Can you work these out from the model? Positions are in its coordinate system, mm. Give positions to 0.01 mm unless a question says otherwise; leave off trailing zeros. Loops run counter-clockwise (first coordinate to the right, second up) from the corner with the lowest first, then second, coordinate; pieces in that order, holes last. Notation, with made-up numbers: M 65.25,79 L 117.25,79 A23 cw 117.25,115 Z; hole C 35,41.5 d5. An arc over 180 degrees is marked long. One line per item, written item: value. Start each with the question number.
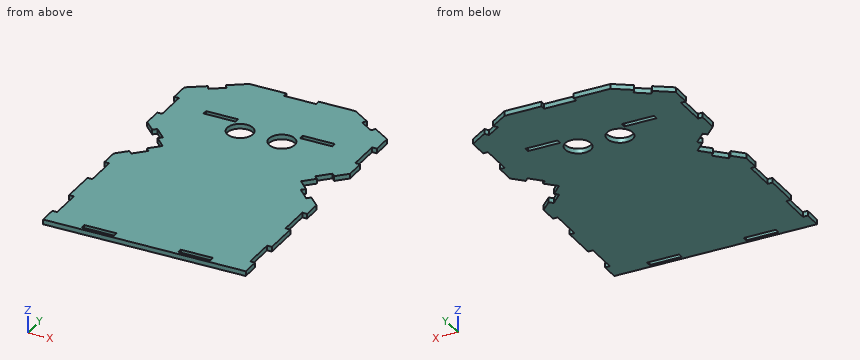
from build123d import *

# Parameters (mm, degrees)
SKETCH1_R           = 8
SKETCH1_W           = 20
SKETCH1_H           = 3
BOSS_EXTRUDE1_DEPTH = 3


with BuildPart() as part:
    # Sketch1 → Boss-Extrude1 (new body)
    with BuildSketch(Plane.XY):
        Polygon((62.274694919, 0), (62.274694919, -11), (59.274694919, -11), (59.274694919, -31), (62.274694919, -31), (62.274694919, -53), (59.274694919, -53), (59.274694919, -73), (62.274694919, -73), (62.274694919, -84), (-63.725305081, -84), (-63.725305081, -73), (-60.725305081, -73), (-60.725305081, -53), (-63.725305081, -53), (-63.725305081, -31), (-60.725305081, -31), (-60.725305081, -11), (-63.725305081, -11), (-63.725305081, 0), (-57.260838987, 6.464466094), (-55.139518643, 4.343145751), (-48.068450831, 11.414213562), (-50.189771175, 13.535533906), (-43.725305081, 20), (-50.189771175, 26.464466094), (-48.068450831, 28.585786438), (-55.139518643, 35.656854249), (-57.260838987, 33.535533906), (-63.725305081, 40), (-63.725305081, 52), (-60.725305081, 52), (-60.725305081, 72), (-63.725305081, 72), (-63.725305081, 84), (-52.885556553, 91.226499019), (-51.221455964, 88.730348136), (-42.90095302, 94.277350098), (-44.565053609, 96.773500981), (-33.725305081, 104), (-10.725305081, 104), (-10.725305081, 101), (9.274694919, 101), (9.274694919, 104), (32.274694919, 104), (43.114443447, 96.773500981), (41.450342859, 94.277350098), (49.770845802, 88.730348136), (51.434946391, 91.226499019), (62.274694919, 84), (62.274694919, 72), (59.274694919, 72), (59.274694919, 52), (62.274694919, 52), (62.274694919, 40), (55.810228825, 33.535533906), (53.688908482, 35.656854249), (46.61784067, 28.585786438), (48.739161013, 26.464466094), (42.274694919, 20), (48.739161013, 13.535533906), (46.61784067, 11.414213562), (53.688908482, 4.343145751), (55.810228825, 6.464466094), align=None)
        with Locations((-13.725305081, 54.688830471)):
            Circle(SKETCH1_R, mode=Mode.SUBTRACT)
        with Locations(Location((12.274694919, 54.688830471, 0), (0, 0, 180))):
            Circle(SKETCH1_R, mode=Mode.SUBTRACT)
        with Locations((29.274694919, -80.5)):
            Rectangle(SKETCH1_W, SKETCH1_H, mode=Mode.SUBTRACT)
        with Locations((-30.725305081, -80.5)):
            Rectangle(SKETCH1_W, SKETCH1_H, mode=Mode.SUBTRACT)
        with Locations((29.274694919, 64.35252343)):
            Rectangle(SKETCH1_W, SKETCH1_H, mode=Mode.SUBTRACT)
        with Locations((-30.725305081, 64.35252343)):
            Rectangle(SKETCH1_W, SKETCH1_H, mode=Mode.SUBTRACT)
    extrude(amount=BOSS_EXTRUDE1_DEPTH)


solid = part.part
Q1. If we section it at A-A, the plane x = -25.5: Write out the boundary of the cut face in (y, z), plus the area to 3 significant figures.
Q2. If we section it at D-D, the plane z = 1.7: Give the number of separate pieces and of enclosed holes in the cut face, plus the area to 3 significant figures.
Q3. If we section it at C-C, the plane y = -71: Write out the boundary of the cut face in (x, z).
Q4. If we section it at B-B, the plane y = 49: Write out the boundary of the cut face in (x, z), plus the area to 3 significant figures.
Q5. I need wall thicknesses on line 1 along Y through (x, z) = (32, 1.7); line 2 along Y through (x, z) = (-34.5, 1.3); line 3 along X through (y, z) = (49.5, 2.65). Which ranges of each line are inside material? Lowest first, please.
Q6. For P1, Ø0.9, axis at y = 66.5, z = 2, coming from the +X side; P2, Ø0.9, axis at y = 64, z = 1.5, coming from the -X side; P3, Ø0.9, axis at x = -62.5, z = 1, coming from the +Y side, each with a flat end and sliding along its axis, tell me the tip position at first contact or that it passes through.
Response:
1. outline: M -84,0 L -82,0 L -82,3 L -84,3 Z; M -79,0 L 62.85,0 L 62.85,3 L -79,3 Z; M 65.85,0 L 104,0 L 104,3 L 65.85,3 Z
1. area: 546 mm^2
2. separate pieces: 1
2. enclosed holes: 6
2. area: 21,000 mm^2
3. outline: M -60.73,0 L 59.27,0 L 59.27,3 L -60.73,3 Z
4. outline: M -63.73,0 L -19.35,0 L -19.35,3 L -63.73,3 Z; M -8.1,0 L 6.65,0 L 6.65,3 L -8.1,3 Z; M 17.9,0 L 62.27,0 L 62.27,3 L 17.9,3 Z
4. area: 311 mm^2
5. line 1: -84 to -82, -79 to 62.85, 65.85 to 104
5. line 2: -84 to -82, -79 to 62.85, 65.85 to 103.48
5. line 3: -63.73 to -19.81, -7.64 to 6.19, 18.36 to 62.27
6. P1: x = 59.27
6. P2: x = -60.73
6. P3: y = 85.12
